Can you work these out from the model? Positions are in its coordinate system, mm. A direction names the side the tool comes from. Round coordinates to 2 decimals unless told otherwise and drop trailing zeros. Write each loop counter-clockwise with the first axis right and the second up, starting at its lowest first coordinate (ties: lowest second). Pieces come first, ordered by that corner, then holes. Notation, with made-up numbers: (-25, 44) -> (28, 44) arc R24 cw to (28, 69) -> close; hole circle Ø7 at (51.25, 45.25). An arc over 180 degrees is marked (long way). Write item = value, one per line. Start each with the question number.
1) Thinking about a two-plate mould opening in X: for faces 1 (the face through (-53.256, 0, 19)), 2 (the face through (-24, -10, 19)), 3 (the face through (-11, -1.85, 19)), 4 (the face through (-5.906, 0, 19)), which applies, +X half, -X half, draft (parallel to the pull), parting line (faces both ways), or undercut?
2) Imagine slicing it at B-B, the plane z = 19.6. Please give me the cut outline in (x, y) (3 decimals).
3) I'm going to push a flat-ended pin straight in: pin 1 (0.8 mm diameter, centred on x = 1.5, y = -0.5, fed in from +Z). Where does the tip first touch, or does it pass through?
4) If I drill on line 1 (Y direction, x = -15, z = 17.4); line 2 (X direction, y = 1.5, z = 19.6), over which ranges is the centre line in solid material (lowest first)?
5) For faces 5 (the face through (-11, 1.85, 19)), 6 (the face through (-24, 0, 17.2)), 7 (the face through (2, 0, 18.2)), which set-ups out of +Z, -Z, +X, -X, +Y, -Y let a thin tool reach every point of the face, with its end or its side?
6) Imagine slicing it at A-A, the plane y = 0. Please give me the cut outline in (x, z), then the cut area to 3 significant figures.
from build123d import *

# Parameters (mm, degrees)
SKETCH_1_W           = 58.5
SKETCH_1_H           = 3
EXTRUDE_1_DEPTH      = 10
EXTRUDE_1_DEPTH_BACK = 10
SKETCH_1_3_W         = 9.7
SKETCH_1_3_H         = 3
CUT_EXTRUDE_1_DEPTH  = 1.85
SKETCH_2_R           = 1.375
CUT_EXTRUDE_2_DEPTH  = 2


with BuildPart() as part:
    # Sketch 1 → Extrude 1 (new body, two sides)
    with BuildSketch(Plane(origin=(0, 0, 0), x_dir=(1, 0, 0), z_dir=(0, 1, 0))) as extrude_1_sk:
        with Locations((-24.00631853, -18.7)):
            Rectangle(SKETCH_1_W, SKETCH_1_H)
    extrude(amount=EXTRUDE_1_DEPTH)
    extrude(extrude_1_sk.sketch, amount=-EXTRUDE_1_DEPTH_BACK)

    # Sketch 1_3 → Cut-Extrude 1 (cut, symmetric)
    with BuildSketch(Plane(origin=(0, 0, 0), x_dir=(1, 0, 0), z_dir=(0, 1, 0))):
        with Locations((-10.75631853, -18.7)):
            Rectangle(SKETCH_1_3_W, SKETCH_1_3_H)
    extrude(amount=CUT_EXTRUDE_1_DEPTH, both=True, mode=Mode.SUBTRACT)

    # Sketch 2 → Cut-Extrude 2 (cut)
    with BuildSketch(Plane.XY.offset(20.2)):
        with Locations((2.24368147, 0)):
            Circle(SKETCH_2_R)
    extrude(amount=-CUT_EXTRUDE_2_DEPTH, mode=Mode.SUBTRACT)


solid = part.part
Reported:
q1.face_1 = -X half
q1.face_2 = draft
q1.face_3 = undercut
q1.face_4 = undercut
q2.outline = (-53.256, -10) -> (5.244, -10) -> (5.244, 10) -> (-53.256, 10) -> close; hole (-15.606, -1.85) -> (-5.906, -1.85) -> (-5.906, 1.85) -> (-15.606, 1.85) -> close; hole circle Ø2.75 at (2.244, 0)
q3.pin_1 = 18.2
q4.line_1 = -10 to -1.85, 1.85 to 10
q4.line_2 = -53.26 to -15.61, -5.91 to 5.24
q5.face_5 = +Z, -Z
q5.face_6 = -Z, +X, -X, +Y, -Y
q5.face_7 = +Z
q6.outline = (-53.26, 17.2) -> (-15.61, 17.2) -> (-15.61, 20.2) -> (-53.26, 20.2) -> close; (-5.91, 17.2) -> (5.24, 17.2) -> (5.24, 20.2) -> (3.62, 20.2) -> (3.62, 18.2) -> (0.87, 18.2) -> (0.87, 20.2) -> (-5.91, 20.2) -> close
q6.area = 141 mm²
